Can you work these out from the drawing? Everything is in mm from the part's minimum corner. Give positions to 0.01 mm unless a question says otherwise; leave off trailing zeros. Write each loop counter-clockwise with the first axis right and the second up, starting at its lowest first coordinate (ties: lowest second). Pieces come first, ordered by that corner, then holes. Notation, with made-up numbers: (-23, -7) -> (5, -7) arc R20 ccw to (5, 32) -> close; hole circle Ø6 at (-16.75, 73). An arc over 180 degrees is marked (long way). Return JSON: item names as keys, results as strings.
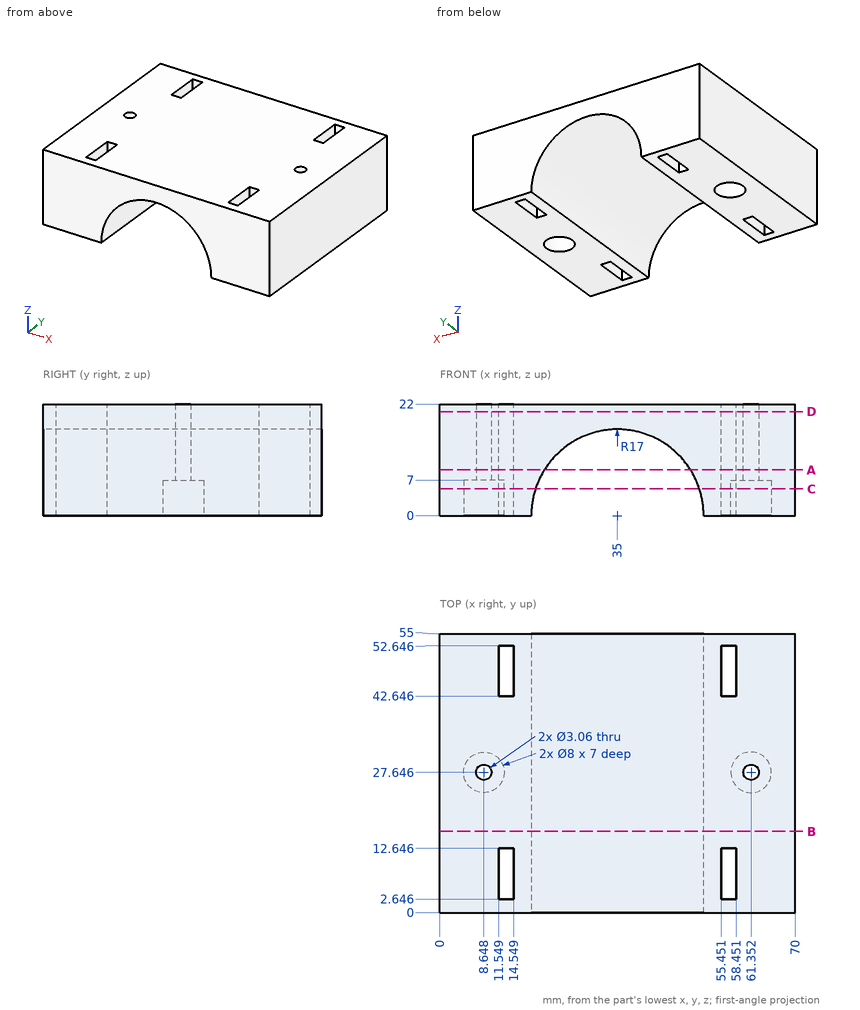
1. If I drill on line 1 (X direction, y = 52.5, z = 18.5); line 2 (Y direction, x = 12, z = 11.5); line 3 (X direction, y = 11.5, z = 5.25), over which ranges is the centre line in solid material (lowest first)? Write a range as [from, to].
Taken from the geometry:
{"line 1": "x = [0, 11.55], [14.55, 55.45], [58.45, 70]", "line 2": "y = [0, 2.65], [12.65, 42.65], [52.65, 55]", "line 3": "x = [0, 11.55], [14.55, 18.83], [51.17, 55.45], [58.45, 70]"}
2. Suppose I cut it at A-A, the plane z = 9. List the corners of the cut face in (x, y) for me.
Taken from the geometry:
{"outline": "(0, 0) -> (20.58, 0) -> (20.58, 55) -> (0, 55) -> close; (49.42, 0) -> (70, 0) -> (70, 55) -> (49.42, 55) -> close; hole circle Ø3.06 at (8.65, 27.65); hole (11.55, 2.65) -> (14.55, 2.65) -> (14.55, 12.65) -> (11.55, 12.65) -> close; hole (11.55, 42.65) -> (14.55, 42.65) -> (14.55, 52.65) -> (11.55, 52.65) -> close; hole (55.45, 2.65) -> (58.45, 2.65) -> (58.45, 12.65) -> (55.45, 12.65) -> close; hole (55.45, 42.65) -> (58.45, 42.65) -> (58.45, 52.65) -> (55.45, 52.65) -> close; hole circle Ø3.06 at (61.35, 27.65)"}
3. Suppose I cut it at C-C, the plane z = 5.25. List the corners of the cut face in (x, y) for me, and give its area (3 significant figures).
Taken from the geometry:
{"outline": "(0, 0) -> (18.83, 0) -> (18.83, 55) -> (0, 55) -> close; (51.17, 0) -> (70, 0) -> (70, 55) -> (51.17, 55) -> close; hole circle Ø8 at (8.65, 27.65); hole (11.55, 2.65) -> (14.55, 2.65) -> (14.55, 12.65) -> (11.55, 12.65) -> close; hole (11.55, 42.65) -> (14.55, 42.65) -> (14.55, 52.65) -> (11.55, 52.65) -> close; hole (55.45, 2.65) -> (58.45, 2.65) -> (58.45, 12.65) -> (55.45, 12.65) -> close; hole (55.45, 42.65) -> (58.45, 42.65) -> (58.45, 52.65) -> (55.45, 52.65) -> close; hole circle Ø8 at (61.35, 27.65)", "area": "1,850 mm²"}
4. Suppose I cut it at D-D, the plane z = 20.5. List the corners of the cut face in (x, y) for me, and give its area (3 significant figures).
Taken from the geometry:
{"outline": "(0, 0) -> (70, 0) -> (70, 55) -> (0, 55) -> close; hole circle Ø3.06 at (8.65, 27.65); hole (11.55, 2.65) -> (14.55, 2.65) -> (14.55, 12.65) -> (11.55, 12.65) -> close; hole (11.55, 42.65) -> (14.55, 42.65) -> (14.55, 52.65) -> (11.55, 52.65) -> close; hole (55.45, 2.65) -> (58.45, 2.65) -> (58.45, 12.65) -> (55.45, 12.65) -> close; hole (55.45, 42.65) -> (58.45, 42.65) -> (58.45, 52.65) -> (55.45, 52.65) -> close; hole circle Ø3.06 at (61.35, 27.65)", "area": "3,720 mm²"}
5. For pin 1 Ø10 at (x, y) = (27.5, 29.5) entering from -Z; pin 2 Ø4 at (x, y) = (35.5, 41.5) entering from -Z (1 decimal); pin 3 Ø6.5 at (x, y) = (61.35, 27.65) entering from -Z, each with a flat end and sliding along its axis, tell me the tip position at first contact or that it passes through.
Taken from the geometry:
{"pin 1": "stops at z = 11.52", "pin 2": "stops at z = 16.8", "pin 3": "stops at z = 7"}
6. Suppose I cut it at B-B, the plane y = 16. List the corners of the cut face in (x, z) for me.
Taken from the geometry:
{"outline": "(0, 0) -> (18, 0) arc R17 cw to (52, 0) -> (70, 0) -> (70, 22) -> (0, 22) -> close"}
